Input: part model. Units: mm. Frame: model coordinates. Face numbers are marked on the shaded views. A direction names the side the tool comes from. Round coordinates to 2 decimals unless told otherwise and drop trailing zeros. Loops run counter-clockwise (first coordinate to the right, second up) from the corner with the lowest first, then second, coordinate; pieces in that order, holes last. Notation, with made-up numbers: (19.5, -14.75) -> (43.5, -14.75) arc R19 ccw to (43.5, 18.25) -> close; hole circle Ø3 at (49, 81.5). An arc over 180 degrees is marked (long way). Answer as a JSON object with one key per item and string values. Group by question number.
Item 1: Material intervals for line 1 (Y direction, x = 9.5, z = 0.7); line 2 (Y direction, x = -9.5, z = 1.65); line 3 (Z direction, x = 0, y = -5.3), sorted ascending. Write a range as [from, to].
Item 2: Section query A-A on x = 0. Count the separate pieces of the cut face and the enclosed holes in it, and give its area (3 significant figures).
Item 3: Pin query (flat end, axial travel): pin 1 (1 mm diameter, centred on y = -0.5, z = -7, fed in from +X); pin 2 (6 mm diameter, centred on x = 0, z = -7, fed in from -Y); pin 3 (2 mm diameter, centred on y = -6.5, z = -7.5, fed in from -X). Return the tip coordinate at first contact, or that it passes through.
Item 4: Section query C-C on z = -6.6. Return loops of the section in (x, y), and give its area (3 significant figures).
Item 5: Section query D-D on z = -2.25. Return loops of the section in (x, y).
Item 6: Set-up query: the marked faces 1, 2, 3, 4 and 5. Return all of +Z, -Z, +X, -X, +Y, -Y with unobstructed straight access to the full face (end or side cutting, diameter ignored); none if empty.
Item 7: Section query B-B on z = -15.5. Return loops of the section in (x, y), and give its area (3 significant figures).
Item 8: Draft query along Y for the marked faces 6, 7, 8 and 9. Return one class per face: released by +Y, released by -Y, zero draft, split by the parting line, or undercut.
from build123d import *

# Parameters (mm, degrees)
SKETCH_R        = 1.75
PAD_DEPTH       = 4.6
SKETCH001_R     = 11
SKETCH001_W     = 16.2
SKETCH001_H     = 8.2
PAD001_DEPTH    = 23
SKETCH002_W     = 16.2
SKETCH002_H     = 8.2
POCKET_DEPTH    = 4.601
SKETCH003_W     = 0.7
SKETCH003_H     = 3.9
SKETCH003_W_2   = 3.9
SKETCH003_H_2   = 0.7
POCKET001_DEPTH = 15.5
FILLET001_R     = 1
SKETCH004_W     = 10.740578
SKETCH004_H     = 1.4
POCKET002_DEPTH = 22
SKETCH005_R     = 1.2
POCKET003_DEPTH = 25.101
SKETCH006_R     = 2.7
POCKET004_DEPTH = 2
CHAMFER_1_ANGLE = 48
CHAMFER_1_SIZE  = 1.5
CHAMFER_2_ANGLE = 48
CHAMFER_2_SIZE  = 1.5
FILLET_R        = 1
CHAMFER001_SIZE = 1


with BuildPart() as part:
    # Sketch → Pad (new body)
    with BuildSketch(Plane.XY):
        with BuildLine():
            Line((-13, 12), (-13, -12))
            ThreePointArc((-13, -12), (-11.974874, -14.474874), (-9.5, -15.5))
            Line((-9.5, -15.5), (9.5, -15.5))
            ThreePointArc((9.5, -15.5), (11.974874, -14.474874), (13, -12))
            Line((13, -12), (13, 12))
            ThreePointArc((13, 12), (11.974874, 14.474874), (9.5, 15.5))
            Line((9.5, 15.5), (-9.5, 15.5))
            ThreePointArc((-9.5, 15.5), (-11.974874, 14.474874), (-13, 12))
        make_face()
        with Locations((-9.5, 12)):
            Circle(SKETCH_R, mode=Mode.SUBTRACT)
        with Locations((9.5, -12)):
            Circle(SKETCH_R, mode=Mode.SUBTRACT)
    extrude(amount=PAD_DEPTH)

    # Sketch001 → Pad001 (join)
    with BuildSketch(Plane(origin=(0, 0, 0), x_dir=(1, 0, 0), z_dir=(0, 0, -1))):
        Circle(SKETCH001_R)
        Rectangle(SKETCH001_W, SKETCH001_H, mode=Mode.SUBTRACT)
    extrude(amount=PAD001_DEPTH)

    # Sketch002 (on Face19 of Pad001) → Pocket (cut, through all)
    with BuildSketch(Plane(origin=(0, 0, 0), x_dir=(1, 0, 0), z_dir=(0, 0, -1))):
        Rectangle(SKETCH002_W, SKETCH002_H)
    extrude(amount=-POCKET_DEPTH, mode=Mode.SUBTRACT)

    # Sketch003 → Pocket001 (cut)
    with BuildSketch(Plane(origin=(0, 0, -23), x_dir=(1, 0, 0), z_dir=(0, 0, -1))):
        with Locations((-8.45, 0)):
            Rectangle(SKETCH003_W, SKETCH003_H)
        with Locations((-3.8, 4.45)):
            Rectangle(SKETCH003_W_2, SKETCH003_H_2)
        with Locations((3.8, 4.45)):
            Rectangle(SKETCH003_W_2, SKETCH003_H_2)
    extrude(amount=-POCKET001_DEPTH, mode=Mode.SUBTRACT)

    # Fillet001
    fillet001_edges = [part.edges().sort_by_distance(p)[0] for p in [
        (-11, 0, -23),
    ]]
    fillet(fillet001_edges, radius=FILLET001_R)

    # Sketch004 (on Face4 of Fillet001) → Pocket002 (cut)
    with BuildSketch(Plane(origin=(0, 0, -23), x_dir=(1, 0, 0), z_dir=(0, 0, -1))):
        with Locations((0, 10.3)):
            Rectangle(SKETCH004_W, SKETCH004_H)
    extrude(amount=-POCKET002_DEPTH, mode=Mode.SUBTRACT)

    # Sketch005 (on Face3 of Pocket002) → Pocket003 (cut, through all)
    with BuildSketch(Plane.XZ.offset(9.6)):
        with Locations((0, -6.6)):
            Circle(SKETCH005_R)
    extrude(amount=-POCKET003_DEPTH, mode=Mode.SUBTRACT)

    # Sketch006 (on Face2 of Pocket003) → Pocket004 (cut)
    with BuildSketch(Plane.XZ.offset(9.6)):
        with Locations((0, -6.6)):
            Circle(SKETCH006_R)
    extrude(amount=-POCKET004_DEPTH, mode=Mode.SUBTRACT)

    # Chamfer 1
    chamfer_1_edges = [part.edges().sort_by_distance(p)[0] for p in [
        (-11.25, 12, 4.6),
    ]]
    chamfer_1_side = part.faces().sort_by_distance((-11.25, 12, 2.3))[0]
    chamfer(chamfer_1_edges, length=CHAMFER_1_SIZE, angle=CHAMFER_1_ANGLE, reference=chamfer_1_side)

    # Chamfer 2
    chamfer_2_edges = [part.edges().sort_by_distance(p)[0] for p in [
        (7.75, -12, 4.6),
    ]]
    chamfer_2_side = part.faces().sort_by_distance((7.75, -12, 2.3))[0]
    chamfer(chamfer_2_edges, length=CHAMFER_2_SIZE, angle=CHAMFER_2_ANGLE, reference=chamfer_2_side)

    # Fillet
    fillet_edges = [part.edges().sort_by_distance(p)[0] for p in [
        (13, 0, 4.6),
        (0, -15.5, 4.6),
        (-13, 0, 4.6),
        (-11.974874, -14.474874, 4.6),
        (11.974874, 14.474874, 4.6),
        (0, 15.5, 4.6),
        (11.974874, -14.474874, 4.6),
        (-11.974874, 14.474874, 4.6),
    ]]
    fillet(fillet_edges, radius=FILLET_R)

    # Chamfer001
    chamfer001_edges = [part.edges().sort_by_distance(p)[0] for p in [
        (0, -4.1, 4.6),
        (-8.1, 0, 4.6),
        (0, 4.1, 4.6),
        (8.1, 0, 4.6),
    ]]
    chamfer(chamfer001_edges, length=CHAMFER001_SIZE)


solid = part.part
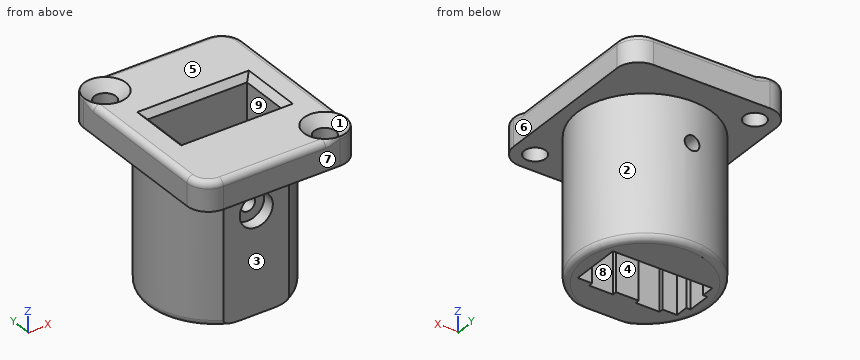
Solved:
{
 "1": {"line 1": "[-15.5, -13.75], [-10.25, 15.5]", "line 2": "[-15.5, 10.25], [13.75, 15.5]", "line 3": "[-23, -7.8], [-5.4, 4.6]"},
 "2": {"separate pieces": "4", "enclosed holes": "0", "area": "354 mm²"},
 "3": {"pin 1": "x = 11", "pin 2": "y = -9.6", "pin 3": "x = -9.53"},
 "4": {"outline": "(-8.1, -4.1) -> (-8.1, 4.1) -> (-1.2, 4.1) -> (-1.2, 10.93) arc R11 ccw to (-5.37, -9.6) -> (-2.7, -9.6) -> (-2.7, -7.6) -> (-1.2, -7.6) -> (-1.2, -4.1) -> close; (1.2, -7.6) -> (2.7, -7.6) -> (2.7, -9.6) -> (5.37, -9.6) arc R11 ccw to (1.2, 10.93) -> (1.2, 4.1) -> (8.1, 4.1) -> (8.1, -4.1) -> (1.2, -4.1) -> close", "area": "201 mm²"},
 "5": {"outline": "(-5.37, -9.6) -> (5.37, -9.6) arc R11 ccw (long way) to start; hole (-8.1, -4.1) -> (8.1, -4.1) -> (8.1, 4.1) -> (-8.1, 4.1) -> close"},
 "6": {"face 1": "+Z", "face 2": "-Z", "face 3": "-Z, +X, -X, -Y", "face 4": "+Z, -Z", "face 5": "+Z, +X, -X, +Y, -Y"},
 "7": {"outline": "(-5.37, -9.6) -> (5.37, -9.6) arc R11 ccw (long way) to start; hole (-8.8, -1.95) -> (-8.1, -1.95) -> (-8.1, -4.1) -> (-5.75, -4.1) -> (-5.75, -4.8) -> (-1.85, -4.8) -> (-1.85, -4.1) -> (1.85, -4.1) -> (1.85, -4.8) -> (5.75, -4.8) -> (5.75, -4.1) -> (8.1, -4.1) -> (8.1, 4.1) -> (-8.1, 4.1) -> (-8.1, 1.95) -> (-8.8, 1.95) -> close", "area": "229 mm²"},
 "8": {"face 6": "zero draft", "face 7": "released by -Y", "face 8": "undercut", "face 9": "undercut"}
}
